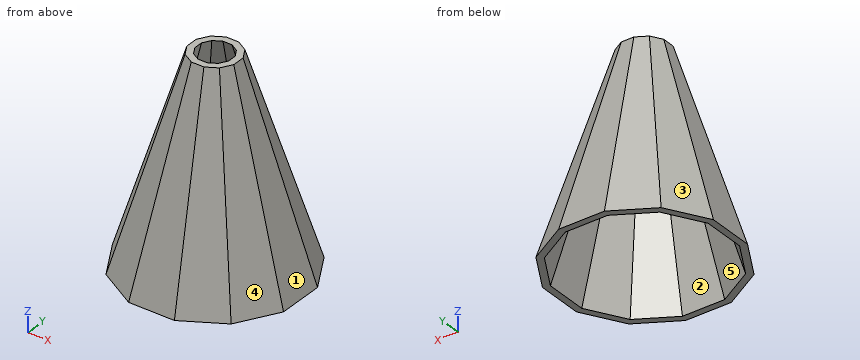
```python
from build123d import *

# Parameters (mm, degrees)
F2_DEPTH = 800
F2_TAPER = 17
F3_T     = 25
F5_DEPTH = 25


with BuildPart() as f2:
    # F0 (on Top) → F2 (new body)
    with BuildSketch(Plane.XY):
        Polygon((-310.8845726812, 83.3012701892), (-310.8845726812, -83.3012701892), (-227.583302492, -227.583302492), (-83.3012701892, -310.8845726812), (83.3012701892, -310.8845726812), (227.583302492, -227.583302492), (310.8845726812, -83.3012701892), (310.8845726812, 83.3012701892), (227.583302492, 227.583302492), (83.3012701892, 310.8845726812), (-83.3012701892, 310.8845726812), (-227.583302492, 227.583302492), align=None)
    extrude(amount=F2_DEPTH, taper=F2_TAPER)

    # F3
    f3_openings = [f2.faces().sort_by_distance(p)[0] for p in [
        (0, 0, 0),
    ]]
    offset(amount=F3_T, openings=f3_openings, kind=Kind.INTERSECTION)

    # F4 (on offset) → F5 (cut)
    with BuildSketch(Plane.XY.offset(800)):
        Polygon((93.3012701892, -25), (93.3012701892, 25), (68.3012701892, 68.3012701892), (25, 93.3012701892), (-25, 93.3012701892), (-68.3012701892, 68.3012701892), (-93.3012701892, 25), (-93.3012701892, -25), (-68.3012701892, -68.3012701892), (-25, -93.3012701892), (25, -93.3012701892), (68.3012701892, -68.3012701892), align=None)
    extrude(amount=F5_DEPTH, mode=Mode.SUBTRACT)


solid = f2.part
```
CAD build for the part. Positions are in the model's coordinates, mm. Face numbers are marked on the shaded views. A direction names the side the tool comes from. Round coordinates to 2 decimals unless told otherwise and drop trailing zeros. Order: outer loops, then holes, each group sorted by start corner. A loop starts at its lowest first (then second) coordinate and runs counter-clockwise, first axis right, second up.
Item 1: Saw through at D-D on x = 115.5. Write the cut outline in (y, z).
Item 2: Probe line 1 along X through (y, z) = (183, 270); line 2 along X through (y, z) = (-115.5, 601); line 3 along Y through (x, z) = (98, 604.5). List the from-to ranges inside material, lowest first.
Item 3: Tool access for the marked faces 1 and 2: list every direction of +Z, -Z, +X, -X, +Y, -Y with a clear straight run to the whole face (end or side of a thin tool).
Item 4: Saw through at B-B on z = 304. Write the cut outline in (x, y).
Item 5: Mould opens along X. For the marked faces 3, 4 and 5 say: pulls with the +X half, pulls with the -X half, needs draft (parallel to the pull), parting line crosses it, or undercut.
Item 6: Saw through at C-C on y = -135.5. Write the cut outline in (x, z), then the cut area to 3 significant figures.
Item 7: Saw through at A-A on y = 2.5. Write the cut outline in (x, z), then the cut area to 3 significant figures.
Item 8: Pin check, flat tips, straight feed: pin 1 (5 mm diameter, centred on y = -55, z = 529.5, fed in from -X); pin 2 (3 mm diameter, centred on x = 10, z = 578.5, fed in from +Y); pin 3 (1 mm diameter, centred on y = -14, z = 315, fed in from -X). Stop position of each tip, or through.
Reported:
1. outline: (-322.48, 0) - (-292.29, 0) - (-115.5, 500.8) - (-30.95, 639.07) - (30.95, 639.07) - (115.5, 500.8) - (292.29, 0) - (322.48, 0) - (115.5, 586.3) - (30.95, 724.58) - (-30.95, 724.58) - (-115.5, 586.3) - close
2. line 1: x = -188.19 to -139.71, 139.71 to 188.19
2. line 2: x = -106.51 to -54.23, 54.23 to 106.51
2. line 3: y = -119.18 to -82.4, 82.4 to 119.18
3. face 1: +Z, +X, +Y, -Y
3. face 2: -Z
4. outline: (-244.08, -65.4) - (-178.68, -178.68) - (-65.4, -244.08) - (65.4, -244.08) - (178.68, -178.68) - (244.08, -65.4) - (244.08, 65.4) - (178.68, 178.68) - (65.4, 244.08) - (-65.4, 244.08) - (-178.68, 178.68) - (-244.08, 65.4) - close; hole (-217.94, -58.4) - (-159.54, -159.54) - (-58.4, -217.94) - (58.4, -217.94) - (159.54, -159.54) - (217.94, -58.4) - (217.94, 58.4) - (159.54, 159.54) - (58.4, 217.94) - (-58.4, 217.94) - (-159.54, 159.54) - (-217.94, 58.4) - close
5. face 3: pulls with the -X half
5. face 4: pulls with the +X half
5. face 5: undercut
6. outline: (-310.93, 0) - (-280.75, 0) - (-135.5, 411.43) - (-36.31, 573.66) - (36.31, 573.66) - (135.5, 411.43) - (280.75, 0) - (310.93, 0) - (135.5, 496.94) - (36.31, 659.16) - (-36.31, 659.16) - (-135.5, 496.94) - close
6. area: 50,600 mm2
7. outline: (-337.03, 0) - (-310.88, 0) - (-66.3, 800) - (-92.44, 800) - close; (66.3, 800) - (310.88, 0) - (337.03, 0) - (92.44, 800) - close
7. area: 41,800 mm2
8. pin 1: stops at x = -172.17
8. pin 2: stops at y = 160.62
8. pin 3: stops at x = -240.87
